```python
from build123d import *

# Parameters (mm, degrees)
BOSS_EXTRUDE1_DEPTH = 5.08
SKETCH2_W           = 101.6
SKETCH2_H           = 10.16
CUT_EXTRUDE3_DEPTH  = 22.86
SKETCH9_R           = 1.27
CUT_EXTRUDE4_DEPTH  = 25.908
SKETCH13_W          = 11.0236
SKETCH13_H          = 5.0038
CUT_EXTRUDE5_DEPTH  = 25.908
SKETCH8_R           = 8.636
CUT_EXTRUDE6_DEPTH  = 25.908
SKETCH14_W          = 212.203069611
SKETCH14_H          = 122.52066239
SKETCH14_W_2        = 52.5744
SKETCH14_H_2        = 29.137232508
CUT_EXTRUDE7_DEPTH  = 25.908
SKETCH15_W          = 52.5744
SKETCH15_H          = 43.722211583
BOSS_EXTRUDE2_DEPTH = 5.08
SKETCH17_W          = 25.579382718
SKETCH17_H          = 36.902767492
CUT_EXTRUDE8_DEPTH  = 10.16
SKETCH18_R          = 1.7526
CUT_EXTRUDE9_DEPTH  = 10.16
SKETCH19_W          = 77.987144431
SKETCH19_H          = 16.36926668
CUT_EXTRUDE10_DEPTH = 19.05
SKETCH20_R          = 1.778
CUT_EXTRUDE11_DEPTH = 19.05


with BuildPart() as part:
    # Sketch1 → Boss-Extrude1 (new body)
    with BuildSketch(Plane(origin=(0, 0, 0), x_dir=(0, 0, -1), z_dir=(1, 0, 0))):
        Polygon((62.997029703, -55.82970297), (88.397029703, -55.82970297), (88.397029703, -65.98970297), (-89.402970297, -65.98970297), (-89.402970297, -55.82970297), (-64.002970297, -55.82970297), (-64.002970297, 27.837475742), (62.997029703, 27.837475742), align=None)
    extrude(amount=BOSS_EXTRUDE1_DEPTH)

    # Sketch2 → Cut-Extrude3 (cut)
    with BuildSketch(Plane(origin=(0, 0, 0), x_dir=(0, 0, -1), z_dir=(1, 0, 0))):
        with Locations((-0.502970297, -60.90970297)):
            Rectangle(SKETCH2_W, SKETCH2_H)
    extrude(amount=CUT_EXTRUDE3_DEPTH, mode=Mode.SUBTRACT)

    # Sketch9 → Cut-Extrude4 (cut)
    with BuildSketch(Plane(origin=(0, 0, 0), x_dir=(0, 0, -1), z_dir=(1, 0, 0))):
        with Locations((-22.010170297, -1.223907747)):
            Circle(SKETCH9_R)
        with Locations(Location((-22.010170297, -18.977232508, 0), (0, 0, 180))):
            Circle(SKETCH9_R)
        with Locations((20.404229703, -18.977232508)):
            Circle(SKETCH9_R)
        with Locations(Location((20.404229703, -1.223907747, 0), (0, 0, 180))):
            Circle(SKETCH9_R)
    extrude(amount=CUT_EXTRUDE4_DEPTH, mode=Mode.SUBTRACT)

    # Sketch13 → Cut-Extrude5 (cut)
    with BuildSketch(Plane(origin=(0, 0, 0), x_dir=(0, 0, -1), z_dir=(1, 0, 0))):
        with Locations((-0.746414126, -2.5019)):
            Rectangle(SKETCH13_W, SKETCH13_H)
    extrude(amount=CUT_EXTRUDE5_DEPTH, mode=Mode.SUBTRACT)

    # Sketch8 → Cut-Extrude6 (cut)
    with BuildSketch(Plane(origin=(0, 0, 0), x_dir=(0, 0, -1), z_dir=(1, 0, 0))):
        with Locations((12.197029703, -10.100570128)):
            Circle(SKETCH8_R)
        with Locations((-13.710970297, -10.100570128)):
            Circle(SKETCH8_R)
    extrude(amount=CUT_EXTRUDE6_DEPTH, mode=Mode.SUBTRACT)

    # Sketch14 → Cut-Extrude7 (cut)
    with BuildSketch(Plane(origin=(0, 0, 0), x_dir=(0, 0, -1), z_dir=(1, 0, 0))):
        with Locations((-5.581398167, -16.698007888)):
            Rectangle(SKETCH14_W, SKETCH14_H)
        with Locations((-0.802970297, -9.488616254)):
            Rectangle(SKETCH14_W_2, SKETCH14_H_2, mode=Mode.SUBTRACT)
    extrude(amount=CUT_EXTRUDE7_DEPTH, mode=Mode.SUBTRACT)

    # Sketch15 → Boss-Extrude2 (add)
    with BuildSketch(Plane(origin=(0, 0, 0), x_dir=(0, 0, -1), z_dir=(1, 0, 0))):
        with Locations((-0.802970297, -44.178894209)):
            Rectangle(SKETCH15_W, SKETCH15_H)
    extrude(amount=BOSS_EXTRUDE2_DEPTH)

    # Sketch17 → Cut-Extrude8 (cut)
    with BuildSketch(Plane(origin=(0, 0, 0), x_dir=(0, 0, -1), z_dir=(1, 0, 0))):
        with Locations((-17.869691359, -42.508616254)):
            Rectangle(SKETCH17_W, SKETCH17_H)
        with Locations((17.869691359, -42.508616254)):
            Rectangle(SKETCH17_W, SKETCH17_H)
    extrude(amount=CUT_EXTRUDE8_DEPTH, mode=Mode.SUBTRACT)

    # Sketch18 → Cut-Extrude9 (cut)
    with BuildSketch(Plane(origin=(0, -66.04, 0), x_dir=(1, 0, 0), z_dir=(0, 1, 0))):
        with Locations((0, -22.010170297)):
            Circle(SKETCH18_R)
        with Locations((0, 20.404229703)):
            Circle(SKETCH18_R)
    extrude(amount=CUT_EXTRUDE9_DEPTH, mode=Mode.SUBTRACT)

    # Sketch19 → Cut-Extrude10 (cut)
    with BuildSketch(Plane(origin=(0, 0, 0), x_dir=(0, 0, -1), z_dir=(1, 0, 0))):
        with Locations((-1.479514925, -60.181865848)):
            Rectangle(SKETCH19_W, SKETCH19_H)
    extrude(amount=CUT_EXTRUDE10_DEPTH, mode=Mode.SUBTRACT)

    # Sketch20 → Cut-Extrude11 (cut)
    with BuildSketch(Plane(origin=(0, 0, 0), x_dir=(0, 0, -1), z_dir=(1, 0, 0))):
        with Locations(Location((0, -48.26, 0), (0, 0, 180))):
            Circle(SKETCH20_R)
        with Locations(Location((0, -35.56, 0), (0, 0, 180))):
            Circle(SKETCH20_R)
    extrude(amount=CUT_EXTRUDE11_DEPTH, mode=Mode.SUBTRACT)


solid = part.part
```
Could you check a few things on this model? Use its own coordinates, in mm. A direction names the side the tool comes from. Round coordinates to 2 decimals unless told otherwise and drop trailing zeros. Write each loop counter-clockwise with the first axis right and the second up, starting at its lowest first coordinate (ties: lowest second). Pieces come first, ordered by that corner, then holes. Notation, with made-up numbers: M 34,18 L 78,18 A17 ccw 78,34 Z; hole C -20.5,8.5 d5. An arc over 180 degrees is marked long. Answer in a Markdown table with one row per item. Add a question column.
Q1. If I drill on line 1 (Y direction, x = 4, z = 0); line 2 (Z direction, x = 4.7, y = -10.5); line 3 (Z direction, x = 3.8, y = -48.26), over which ranges is the centre line in solid material (lowest first)? Write a range as from..to.
Q2. Imagine slicing it at D-D (z = 20). Please give me the cut outline in (x, y).
Q3. Imagine slicing it at A-A (z = 0). Please give me the cut outline in (x, y), then the cut area to 3 significant figures.
Q4. Imagine slicing it at C-C (y = -9). Please give me the cut outline in (x, z).
Q5. Imagine slicing it at B-B (y = -35.56). Please give me the cut outline in (x, z), then the cut area to 3 significant figures.
Q6. Will these pins go through, and if not, where does the flat tip stop? pin 1 Ø3.5 at (y, z) = (-18.98, -20.4) entering from +X; pin 2 Ø2.5 at (x, y) = (2.5, -40) entering from -Z; pin 3 Ø1.5 at (x, z) = (3.5, 20) entering from -Y; pin 4 Ø2.5 at (x, y) = (1.5, -44.5) entering from +Z.
Q7. On a 3-axis mill with a long thin cutter (end or side, diameter ignored), from which of +Z, -Z, +X, -X, +Y, -Y can I reach the whole of each face in a straight line? I mean faces 4 (the flat face through (3, -5.004, 1)), 5 (the flat face through (3, -38, -5.08)), 6 (the flat face through (3, -38, 5.08)). Say none if no direction works.
Q8. If we mould it in two halves opening along Z, with no side actions, what happens to faces 1 (the flat face through (3, -10, -25.484)), 2 (the flat face through (0, -17, 1)), 3 (the cylindrical face through (2.5, -1.54, 14.84))? For each: +Z half, -Z half, draft (parallel to the pull), parting line (faces both ways), or undercut.
Values:
| question | item | result |
|---|---|---|
| 1 | line 1 | -52..-50.04, -46.48..-37.34, -33.78..-5, 0..5.08 |
| 1 | line 2 | -25.48..-20.82, -3.57..5.08, 22.34..27.09 |
| 1 | line 3 | -5.08..-1.78, 1.78..5.08 |
| 2 | outline | M 0,-24.06 L 5.08,-24.06 L 5.08,-16.02 L 0,-16.02 Z; M 0,-4.18 L 5.08,-4.18 L 5.08,5.08 L 0,5.08 Z |
| 3 | outline | M 0,-52 L 5.08,-52 L 5.08,-50.04 L 0,-50.04 Z; M 0,-46.48 L 5.08,-46.48 L 5.08,-37.34 L 0,-37.34 Z; M 0,-33.78 L 5.08,-33.78 L 5.08,-5 L 0,-5 Z; M 0,0 L 5.08,0 L 5.08,5.08 L 0,5.08 Z |
| 3 | area | 228 mm^2 |
| 4 | outline | M 0,-25.48 L 5.08,-25.48 L 5.08,-20.76 L 0,-20.76 Z; M 0,-3.63 L 5.08,-3.63 L 5.08,5.15 L 0,5.15 Z; M 0,22.28 L 5.08,22.28 L 5.08,27.09 L 0,27.09 Z |
| 5 | outline | M 0,-5.08 L 5.08,-5.08 L 5.08,-1.78 L 0,-1.78 Z; M 0,1.78 L 5.08,1.78 L 5.08,5.08 L 0,5.08 Z |
| 5 | area | 33.5 mm^2 |
| 6 | pin 1 | x = 5.08 |
| 6 | pin 2 | z = -5.08 |
| 6 | pin 3 | y = -24.06 |
| 6 | pin 4 | z = 5.08 |
| 7 | face 4 | +X, -X |
| 7 | face 5 | -Z, +X, -X, -Y |
| 7 | face 6 | +Z, +X, -X, -Y |
| 8 | face 1 | -Z half |
| 8 | face 2 | draft |
| 8 | face 3 | undercut |
